```python
from build123d import *

# Parameters (mm, degrees)
F0_W     = 73.66
F0_H     = 98.425
F1_DEPTH = 3.175
F3_DEPTH = 12.7


with BuildPart() as f1:
    # F0 (on Right) → F1 (new body)
    with BuildSketch(Plane.YZ):
        Rectangle(F0_W, F0_H)
    extrude(amount=-F1_DEPTH)

    # F2 (on Front) → F3 (join)
    with BuildSketch(Plane.XZ):
        with BuildLine():
            Line((0, -29.845), (0, -33.02))
            ThreePointArc((0, -33.02), (7.62, -25.4), (0, -17.78))
            Line((0, -17.78), (0, -20.955))
            ThreePointArc((0, -20.955), (4.445, -25.4), (0, -29.845))
        make_face()
    extrude(amount=-F3_DEPTH)


solid = f1.part
```
The listing builds one solid part. Answer for the finished solid, in the listing's coordinates (mm). A direction names the side the tool comes from. Coordinates: 2 decimals unless noted, no trailing zeros. Loops run counter-clockwise (first coordinate to the right, second up) from the corner with the lowest first, then second, coordinate; pieces in that order, holes last. Notation, with made-up numbers: M 85,-23 L 99,-23 A30 ccw 99,9 Z; hole C 3,54.25 d4. An arc over 180 degrees is marked long. Answer as a JSON object with one key per item and string values. Group by question number.
Item 1: Consider L1, parallel to X at y = -20.5, z = -16 (3 decimals); L2, parallel to Z at x = 4, y = 3.5; L3, parallel to Z at x = 1.5, y = 10.5. Determine where each line is inside the solid, lowest interval first.
Item 2: Section B-B (y = 2) is taken. Write down the section's boundary in (x, z) (1 decimal).
Item 3: Section D-D (z = 34) is taken. Write down the section's boundary in (x, y) (3 decimals), and give its area (3 significant figures).
Item 4: Each of these flat-tipped pins is pushed along its axis until it touches: P1, Ø1, axis at y = 3.5, z = 8, coming from the +X side; P2, Ø6, axis at x = 2, z = 2, coming from the +Y side; P3, Ø3, axis at x = 5, y = 10.5, coming from the -Z side; P4, Ø6, axis at x = 5, z = -24, coming from the +Y side. Where does it stop, or does it pass through?
Item 5: Section C-C (y = 24) is taken. Write down the section's boundary in (x, z) (1 decimal).
Item 6: Determine the mould class of faces 3 (the face through (-2, -1, 49.212)), 4 (the face through (4.444, 6.261, -25.302)), 5 (the face through (-2, -1, -49.212)), 6 (the face through (5, 0, -25)) for opening direction Z: +Z half, -Z half, draft (parallel to the pull), parting line (faces both ways), or undercut.
Item 7: Section A-A (z = -25.4) is taken. Write down the section's boundary in (x, y) (3 decimals).
Item 8: Which of the six approach directions +Z, -Z, +X, -X, +Y, -Y give full straight-line access (tool end or side, diameter ignored) to faces 1 (the face through (5, 12.7, -25)), 2 (the face through (-2, 36.83, -1))?
Solved:
{
 "1": {"L1": "x = -3.175 to 0", "L2": "z = -31.89 to -27.34, -23.46 to -18.91", "L3": "z = -32.87 to -29.58, -21.22 to -17.93"},
 "2": {"outline": "M -3.2,-49.2 L 0,-49.2 L 0,-33 A7.6 ccw 0,-17.8 L 0,49.2 L -3.2,49.2 Z; hole M 0,-29.8 A4.4 ccw 0,-21 Z"},
 "3": {"outline": "M -3.175,-36.83 L 0,-36.83 L 0,36.83 L -3.175,36.83 Z", "area": "234 mm2"},
 "4": {"P1": "stops at x = 0", "P2": "stops at y = 36.83", "P3": "stops at z = -32.17", "P4": "stops at y = 12.7"},
 "5": {"outline": "M -3.2,-49.2 L 0,-49.2 L 0,49.2 L -3.2,49.2 Z"},
 "6": {"face 3": "+Z half", "face 4": "undercut", "face 5": "-Z half", "face 6": "draft"},
 "7": {"outline": "M -3.175,-36.83 L 0,-36.83 L 0,36.83 L -3.175,36.83 Z; M 4.445,0 L 7.62,0 L 7.62,12.7 L 4.445,12.7 Z"},
 "8": {"face 1": "+Z, -Z, +X, +Y", "face 2": "+Z, -Z, +X, -X, +Y"}
}
